Source: three-view drawing plus pictorial views. Frame: mm from the lowest corner of the part. A direction names the side the tool comes from. Coordinates: 2 decimals unless noted, no trailing zeros. Write each loop counter-clockwise with the first axis right and the second up, starting at its lowest first coordinate (ties: lowest second). Pieces come first, ordered by that corner, then holes. Notation, with made-up numbers: M 34,80 L 85,80 A25 cw 85,116 Z; hole C -15.75,33 d8. An arc over 180 degrees is marked long. Answer as a JSON object with one key per item and string values. Group by question number.
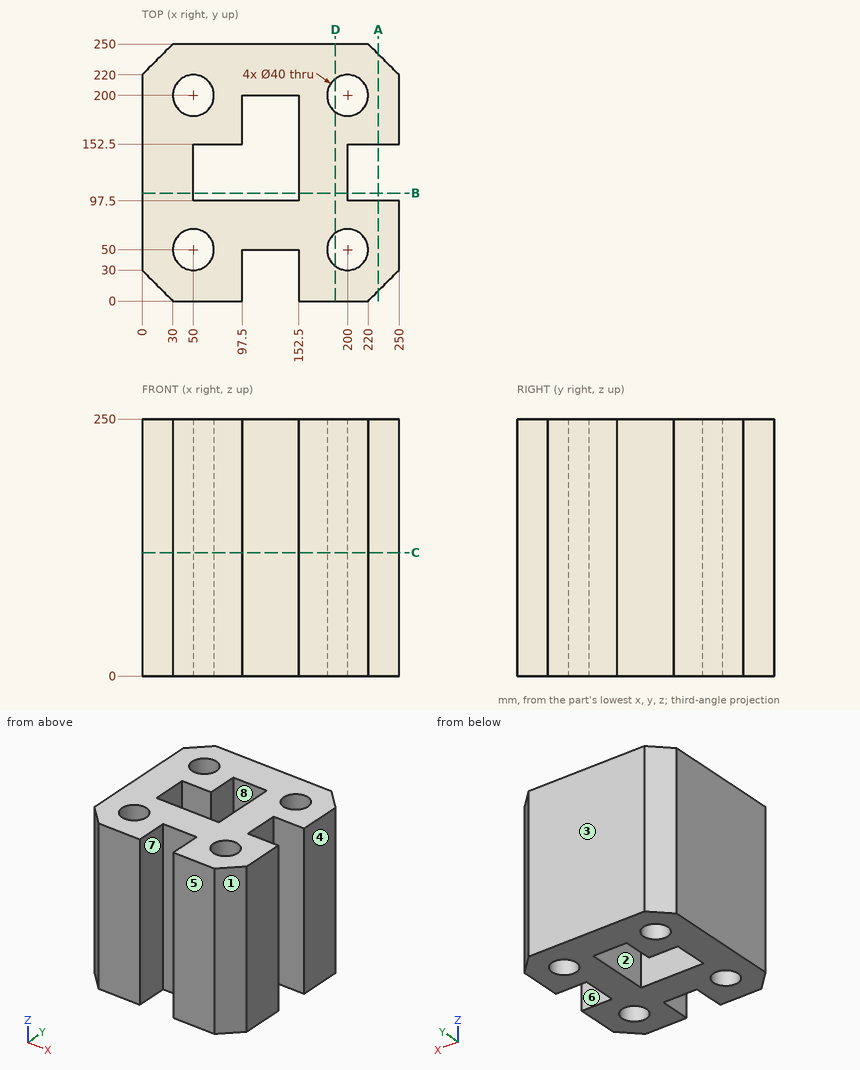
Q1. Draft query along Y for the marked faces 1, 2, 3 and 4. Return one class per face: released by +Y, released by -Y, zero draft, split by the parting line, or undercut.
Q2. Section B-B, the plane y = 105. Return the cut outline in (x, z), and give its area (3 significant figures).
Q3. Section A-A, the plane x = 230. Return the cut outline in (y, z).
Q4. Section D-D, the plane x = 188. Return the cut outline in (y, z).
Q5. Line query: line 1 (X direction, y = 217, z = 143); line 2 (Y direction, x = 65, z = 57); line 3 (X direction, y = 209.5, z = 74). Output: solid intervals per line, ascending. Write a range as from..to.
Q6. Section C-C, the plane z = 120. Return the cut outline in (x, y).
Q7. Access query for the marked faces 5, 6, 7 and 8. Directions: +Z, -Z, +X, -X, +Y, -Y. A direction counts if a zero-diameter tool reaches every point of the face in a straight line with its end or side. Return the directions, or none.
Filled in:
{
 "1": {"face 1": "released by -Y", "face 2": "undercut", "face 3": "released by +Y", "face 4": "zero draft"},
 "2": {"outline": "M 0,0 L 50,0 L 50,250 L 0,250 Z; M 152.5,0 L 200,0 L 200,250 L 152.5,250 Z", "area": "24,400 mm^2"},
 "3": {"outline": "M 10,0 L 97.5,0 L 97.5,250 L 10,250 Z; M 152.5,0 L 240,0 L 240,250 L 152.5,250 Z"},
 "4": {"outline": "M 0,0 L 34,0 L 34,250 L 0,250 Z; M 66,0 L 184,0 L 184,250 L 66,250 Z; M 216,0 L 250,0 L 250,250 L 216,250 Z"},
 "5": {"line 1": "0..39.46, 60.54..189.46, 210.54..250", "line 2": "0..36.77, 63.23..97.5, 152.5..186.77, 213.23..250", "line 3": "0..32.4, 67.6..182.4, 217.6..250"},
 "6": {"outline": "M 0,30 L 30,0 L 97.5,0 L 97.5,50 L 152.5,50 L 152.5,0 L 220,0 L 250,30 L 250,97.5 L 200,97.5 L 200,152.5 L 250,152.5 L 250,220 L 220,250 L 30,250 L 0,220 Z; hole C 50,50 d40; hole C 50,200 d40; hole M 50,97.5 L 152.5,97.5 L 152.5,200 L 97.5,200 L 97.5,152.5 L 50,152.5 Z; hole C 200,50 d40; hole C 200,200 d40"},
 "7": {"face 5": "+Z, -Z, +X, -X, -Y", "face 6": "+Z, -Z, +X", "face 7": "+Z, -Z, -Y", "face 8": "+Z, -Z"}
}
